Source: CAD feature listing. Evaluate the final solid. Frame: model axes, mm. A direction names the side the tool comes from. Coordinates: 2 decimals unless noted, no trailing zeros. Order: outer loops, then holes, each group sorted by start corner. A loop starts at its lowest first (then second) coordinate and runs counter-clockwise, first axis right, second up. Notation, with made-up numbers: (59.25, -23) -> (77.25, -23) arc R21 ccw to (77.25, -15) -> close; hole circle Ø2 at (-32.5, -12). An arc over 180 degrees is marked (long way). Put each result on its own line as item: value.
from build123d import *

# Parameters (mm, degrees)
SKETCH1_W           = 150
SKETCH1_H           = 54
BOSS_EXTRUDE1_DEPTH = 3
SKETCH2_W           = 30
SKETCH2_H           = 35
CUT_EXTRUDE1_DEPTH  = 160.452187191
SKETCH4_W           = 12
SKETCH4_H           = 19
CUT_EXTRUDE2_DEPTH  = 3
SKETCH5_R           = 1.5
CUT_EXTRUDE3_DEPTH  = 3
SKETCH7_R           = 3
CUT_EXTRUDE5_DEPTH  = 1.6
SKETCH8_R           = 1.75
CUT_EXTRUDE6_DEPTH  = 3


with BuildPart() as part:
    # Sketch1 → Boss-Extrude1 (new body)
    with BuildSketch(Plane.XY):
        with Locations((75, 27)):
            Rectangle(SKETCH1_W, SKETCH1_H)
    extrude(amount=BOSS_EXTRUDE1_DEPTH)

    # Sketch2 → Cut-Extrude1 (cut, through all)
    with BuildSketch(Plane(origin=(0, 0, 0), x_dir=(-1, 0, 0), z_dir=(0, 0, -1))):
        with Locations((-15, 17.5)):
            Rectangle(SKETCH2_W, SKETCH2_H)
        with Locations((-135, 17.5)):
            Rectangle(SKETCH2_W, SKETCH2_H)
    extrude(amount=-CUT_EXTRUDE1_DEPTH, mode=Mode.SUBTRACT)

    # Sketch4 → Cut-Extrude2 (cut)
    with BuildSketch(Plane(origin=(0, 0, 0), x_dir=(-1, 0, 0), z_dir=(0, 0, -1))):
        with Locations((-144, 44.5)):
            Rectangle(SKETCH4_W, SKETCH4_H)
        with Locations((-6, 44.5)):
            Rectangle(SKETCH4_W, SKETCH4_H)
    extrude(amount=-CUT_EXTRUDE2_DEPTH, mode=Mode.SUBTRACT)

    # Sketch5 → Cut-Extrude3 (cut)
    with BuildSketch(Plane(origin=(0, 0, 0), x_dir=(-1, 0, 0), z_dir=(0, 0, -1))):
        with Locations((-130, 50)):
            Circle(SKETCH5_R)
        with Locations((-105, 2.5)):
            Circle(SKETCH5_R)
        with Locations(Location((-45, 2.5, 0), (0, 0, 180))):
            Circle(SKETCH5_R)
        with Locations(Location((-20, 50, 0), (0, 0, 180))):
            Circle(SKETCH5_R)
    extrude(amount=-CUT_EXTRUDE3_DEPTH, mode=Mode.SUBTRACT)

    # Sketch7 → Cut-Extrude5 (cut)
    with BuildSketch(Plane.XY.offset(3)):
        with Locations((45, 2.5)):
            Circle(SKETCH7_R)
        with Locations((105, 2.5)):
            Circle(SKETCH7_R)
    extrude(amount=-CUT_EXTRUDE5_DEPTH, mode=Mode.SUBTRACT)

    # Sketch8 → Cut-Extrude6 (cut)
    with BuildSketch(Plane.XY.offset(3)):
        with Locations((30.08, 50.8)):
            Circle(SKETCH8_R)
        with Locations((60.56, 45.72)):
            Circle(SKETCH8_R)
        with Locations((60.5, 17.84)):
            Circle(SKETCH8_R)
        with Locations((36.43, 2.5)):
            Circle(SKETCH8_R)
        with Locations((111.36, 2.5)):
            Circle(SKETCH8_R)
        with Locations((112.63, 50.8)):
            Circle(SKETCH8_R)
    extrude(amount=-CUT_EXTRUDE6_DEPTH, mode=Mode.SUBTRACT)


solid = part.part
1. Cut plane D-D on y = 7. Output: boundary loops of the cut face in (x, z), plus the area to 3 significant figures.
Numbers:
outline: (30, 0) -> (120, 0) -> (120, 3) -> (30, 3) -> close
area: 270 mm2
2. Ray query, line 1 along Y through (x, z) = (45, 0.3); line 2 along Y through (x, z) = (60.56, 1.95); line 3 along X through (y, z) = (4, 2.45). Return the intervals inside material, ascending.
Numbers:
line 1: y = 0 to 1, 4 to 54
line 2: y = 0 to 16.09, 19.59 to 43.97, 47.47 to 54
line 3: x = 30 to 35.53, 37.33 to 42.4, 47.6 to 102.4, 107.6 to 110.46, 112.26 to 120
3. Cut plane A-A on x = 36.43. Output: boundary loops of the cut face in (y, z).
Numbers:
outline: (0, 0) -> (0.75, 0) -> (0.75, 3) -> (0, 3) -> close; (4.25, 0) -> (54, 0) -> (54, 3) -> (4.25, 3) -> close
4. Set-up query: faces 5 (the flat face through (104, 4, 1.4)), 6 (the cylindrical face through (106.5, 2.57, 0.69)). Return all of +Z, -Z, +X, -X, +Y, -Y with unobstructed straight access to the full face (end or side cutting, diameter ignored); none if empty.
Numbers:
face 5: +Z
face 6: +Z, -Z
5. Cut plane C-C on x = 112. Output: boundary loops of the cut face in (y, z), plus the area to 3 significant figures.
Numbers:
outline: (0, 0) -> (0.87, 0) -> (0.87, 3) -> (0, 3) -> close; (4.13, 0) -> (49.17, 0) -> (49.17, 3) -> (4.13, 3) -> close; (52.43, 0) -> (54, 0) -> (54, 3) -> (52.43, 3) -> close
area: 142 mm2
6. Cut plane B-B on z = 0.55. Count the separate pieces of the cut face and the enclosed holes in it, plus the area to 3 significant figures.
Numbers:
separate pieces: 1
enclosed holes: 10
area: 5,460 mm2
7. Pull-direction query (X, two-part tool) for faces 1 (the flat face through (30, 17, 1)), 2 (the cylindrical face through (62.169, 18.366, 1.521)), 3 (the cylindrical face through (19.675, 51.464, 1.479)), 4 (the flat face through (74, 0, 1)); classes: pulls with the +X half, pulls with the -X half, needs draft (parallel to the pull), parting line crosses it, or undercut.
Numbers:
face 1: pulls with the -X half
face 2: undercut
face 3: undercut
face 4: needs draft
8. First-contact query: pin 1 (5 mm diameter, centred on x = 130, y = 50, fed in from +Z); pin 2 (1.6 mm diameter, centred on x = 45.5, y = 4, fed in from +Z); pin 3 (2 mm diameter, centred on x = 111.36, y = 2.5, fed in from -Z); pin 4 (1.5 mm diameter, centred on y = 21, z = 1.5, fed in from +X). Flat tips, straight axial feed; report the tip coordinate or a pass-through.
Numbers:
pin 1: stops at z = 3
pin 2: stops at z = 1.4
pin 3: passes through
pin 4: stops at x = 120
